Verification items for the finished model (mm, model axes). Face numbers are marked on the shaded views. Round coordinates to 2 decimals unless told otherwise and drop trailing zeros. Write each loop counter-clockwise with the first axis right and the second up, starting at its lowest first coordinate (ties: lowest second). Pieces come first, ordered by that corner, then holes. Notation, with made-up numbers: M 3.25,48 L 10.25,48 A12 cw 10.25,69 Z; hole C 78.5,18.25 d8. An arc over 180 degrees is marked long. One line per item, written item: value. Start each with the question number.
from build123d import *

# Parameters (mm, degrees)
F1_DEPTH      = 2
F3_DEPTH      = 2.2
F5_DEPTH      = 25
F6_R          = 1.5
F7_DEPTH      = 4.2
F8_R          = 2.75
F9_DEPTH      = 2
F10_S5_R      = 1.5
F10_T6_DEPTH  = 5
F10_S11_R     = 1.5
F10_T12_DEPTH = 5
F10_S17_R     = 1.5
F10_T18_DEPTH = 5
F10_S23_R     = 1.5
F10_T24_DEPTH = 5
F11_W         = 5.6
F11_H         = 2
F12_DEPTH     = 0.6
F13_T1_DEPTH  = 8.4722813233
F13_T3_DEPTH  = 8.4722813233
F14_SIZE      = 0.5


# Not quite as in the source:
# - a fillet or chamfer that OpenCascade refuses, or shapes differently, is made with other operations: its cross-section is extruded or revolved along the edge and cut away or added


with BuildPart() as f1:
    # F0 (on Top) → F1 (new body)
    with BuildSketch(Plane.XY):
        with BuildLine():
            Line((80, 0), (2, 0))
            ThreePointArc((2, 0), (0.5857864376, -0.5857864376), (0, -2))
            Line((0, -2), (0, -88))
            ThreePointArc((0, -88), (0.5857864376, -89.4142135624), (2, -90))
            Line((2, -90), (11.25, -90))
            Line((11.25, -90), (11.25, -62.5))
            Line((11.25, -62.5), (15.8564011104, -56.3307127986))
            ThreePointArc((15.8564011104, -56.3307127986), (16.5951030311, -54.9153368199), (16.85, -53.3392666362))
            Line((16.85, -53.3392666362), (16.85, -26))
            ThreePointArc((16.85, -26), (17.4357864376, -24.5857864376), (18.85, -24))
            Line((18.85, -24), (63.15, -24))
            ThreePointArc((63.15, -24), (64.5642135624, -24.5857864376), (65.15, -26))
            Line((65.15, -26), (65.15, -53.3392666362))
            ThreePointArc((65.15, -53.3392666362), (65.4048969689, -54.9153368199), (66.1435988896, -56.3307127986))
            Line((66.1435988896, -56.3307127986), (70.75, -62.5))
            Line((70.75, -62.5), (70.75, -90))
            Line((70.75, -90), (80, -90))
            ThreePointArc((80, -90), (81.4142135624, -89.4142135624), (82, -88))
            Line((82, -88), (82, -2))
            ThreePointArc((82, -2), (81.4142135624, -0.5857864376), (80, 0))
        make_face()
    extrude(amount=F1_DEPTH)

    # F2 (on face) → F3 (join)
    with BuildSketch(Plane(origin=(0, 0, 0), x_dir=(1, 0, 0), z_dir=(0, 0, -1))):
        with BuildLine():
            ThreePointArc((80, 0), (81.4142135624, 0.5857864376), (82, 2))
            Line((82, 2), (82, 88))
            ThreePointArc((82, 88), (81.4142135624, 89.4142135624), (80, 90))
            Line((80, 90), (70.75, 90))
            Line((70.75, 90), (70.75, 62.5))
            Line((70.75, 62.5), (70.75, 26))
            ThreePointArc((70.75, 26), (70.1642135624, 24.5857864376), (68.75, 24))
            Line((68.75, 24), (65.15, 24))
            Line((65.15, 24), (16.85, 24))
            Line((16.85, 24), (13.25, 24))
            ThreePointArc((13.25, 24), (11.8357864376, 24.5857864376), (11.25, 26))
            Line((11.25, 26), (11.25, 62.5))
            Line((11.25, 62.5), (11.25, 90))
            Line((11.25, 90), (2, 90))
            ThreePointArc((2, 90), (0.5857864376, 89.4142135624), (0, 88))
            Line((0, 88), (0, 2))
            ThreePointArc((0, 2), (0.5857864376, 0.5857864376), (2, 0))
            Line((2, 0), (80, 0))
        make_face()
    extrude(amount=F3_DEPTH)

    # F4 (on face) → F5 (cut)
    with BuildSketch(Plane.XY.offset(2)):
        with BuildLine():
            Line((18.3, -2), (10.5, -2))
            Line((10.5, -2), (10.5, -7.6))
            ThreePointArc((10.5, -7.6), (11.0857864376, -9.0142135624), (12.5, -9.6))
            Line((12.5, -9.6), (16.3, -9.6))
            ThreePointArc((16.3, -9.6), (17.7142135624, -9.0142135624), (18.3, -7.6))
            Line((18.3, -7.6), (18.3, -2))
        make_face()
    extrude(amount=-F5_DEPTH, mode=Mode.SUBTRACT)

    # F6 (on face) → F7 (cut)
    with BuildSketch(Plane.XY.offset(2)):
        with Locations((5.5, -84.5)):
            Circle(F6_R)
        with Locations((76.5, -84.5)):
            Circle(F6_R)
        with Locations((5.5, -5.5)):
            Circle(F6_R)
        with Locations((76.5, -5.5)):
            Circle(F6_R)
    extrude(amount=-F7_DEPTH, mode=Mode.SUBTRACT)

    # F8 (on face) → F9 (cut)
    with BuildSketch(Plane.XY.offset(2)):
        with Locations((5.5, -5.5)):
            Circle(F8_R)
        with Locations((76.5, -5.5)):
            Circle(F8_R)
        with Locations((76.5, -84.5)):
            Circle(F8_R)
        with Locations((5.5, -84.5)):
            Circle(F8_R)
    extrude(amount=-F9_DEPTH, mode=Mode.SUBTRACT)

    # F10: chamfer of 1.5 on 4 edges, made by hand


with BuildPart() as f10_tool2:
    # F10_s3 → F10_t4 (revolve)
    with BuildSketch(Plane.XZ.offset(84.5)):
        Polygon((8.25, 1.5), (6.75, 0), (8.25, 0), align=None)
    revolve(axis=Axis((5.5, -84.5, 0), (0, 0, 1)))

    # F10_s5 → F10_t6 (cut, symmetric)
    with BuildSketch(Plane.XY.offset(0.7)):
        with Locations((5.5, -84.5)):
            Circle(F10_S5_R)
    extrude(amount=F10_T6_DEPTH, both=True, mode=Mode.SUBTRACT)


with BuildPart() as f1_1:
    add(f1.part)

    # F10_t1: union F10_tool2
    add(f10_tool2.part)


with BuildPart() as f10_tool8:
    # F10_s9 → F10_t10 (revolve)
    with BuildSketch(Plane.XZ.offset(84.5)):
        Polygon((79.25, 1.5), (77.75, 0), (79.25, 0), align=None)
    revolve(axis=Axis((76.5, -84.5, 0), (0, 0, 1)))

    # F10_s11 → F10_t12 (cut, symmetric)
    with BuildSketch(Plane.XY.offset(0.7)):
        with Locations((76.5, -84.5)):
            Circle(F10_S11_R)
    extrude(amount=F10_T12_DEPTH, both=True, mode=Mode.SUBTRACT)


with BuildPart() as f1_2:
    add(f1_1.part)

    # F10_t7: union F10_tool8
    add(f10_tool8.part)


with BuildPart() as f10_tool14:
    # F10_s15 → F10_t16 (revolve)
    with BuildSketch(Plane.XZ.offset(5.5)):
        Polygon((8.25, 1.5), (6.75, 0), (8.25, 0), align=None)
    revolve(axis=Axis((5.5, -5.5, 0), (0, 0, 1)))

    # F10_s17 → F10_t18 (cut, symmetric)
    with BuildSketch(Plane.XY.offset(0.7)):
        with Locations((5.5, -5.5)):
            Circle(F10_S17_R)
    extrude(amount=F10_T18_DEPTH, both=True, mode=Mode.SUBTRACT)


with BuildPart() as f1_3:
    add(f1_2.part)

    # F10_t13: union F10_tool14
    add(f10_tool14.part)


with BuildPart() as f10_tool20:
    # F10_s21 → F10_t22 (revolve)
    with BuildSketch(Plane.XZ.offset(5.5)):
        Polygon((79.25, 1.5), (77.75, 0), (79.25, 0), align=None)
    revolve(axis=Axis((76.5, -5.5, 0), (0, 0, 1)))

    # F10_s23 → F10_t24 (cut, symmetric)
    with BuildSketch(Plane.XY.offset(0.7)):
        with Locations((76.5, -5.5)):
            Circle(F10_S23_R)
    extrude(amount=F10_T24_DEPTH, both=True, mode=Mode.SUBTRACT)


with BuildPart() as f1_4:
    add(f1_3.part)

    # F10_t19: union F10_tool20
    add(f10_tool20.part)

    # F11 (on face) → F12 (join)
    with BuildSketch(Plane(origin=(0, 0, 0), x_dir=(1, 0, 0), z_dir=(0, 0, -1))):
        with Locations((14.05, 43.5)):
            Rectangle(F11_W, F11_H)
        with Locations((67.95, 43.5)):
            Rectangle(F11_W, F11_H)
    extrude(amount=F12_DEPTH)

    # F13: fillet of radius 1.4 on 4 edges, made by hand

    # F13_s2 → F13_t1 (cut)
    with BuildSketch(Plane.YZ.offset(11.25)):
        with BuildLine():
            ThreePointArc((-42.5, 0), (-43.0008384595, -0.4409673646), (-43.6489125293, -0.6))
            Line((-43.6489125293, -0.6), (-42.5, -0.6))
            Line((-42.5, -0.6), (-42.5, 0))
        make_face()
        with BuildLine():
            ThreePointArc((-43.3510874707, -0.6), (-43.9991615405, -0.4409673646), (-44.5, 0))
            Line((-44.5, 0), (-44.5, -0.6))
            Line((-44.5, -0.6), (-43.3510874707, -0.6))
        make_face()
    extrude(amount=F13_T1_DEPTH, mode=Mode.SUBTRACT)

    # F13_s4 → F13_t3 (cut)
    with BuildSketch(Plane.YZ.offset(62.2777186767)):
        with BuildLine():
            ThreePointArc((-43.6489125293, -0.6), (-43.0008384595, -0.4409673646), (-42.5, 0))
            Line((-42.5, 0), (-42.5, -0.6))
            Line((-42.5, -0.6), (-43.6489125293, -0.6))
        make_face()
        with BuildLine():
            ThreePointArc((-44.5, 0), (-43.9991615405, -0.4409673646), (-43.3510874707, -0.6))
            Line((-43.3510874707, -0.6), (-44.5, -0.6))
            Line((-44.5, -0.6), (-44.5, 0))
        make_face()
    extrude(amount=F13_T3_DEPTH, mode=Mode.SUBTRACT)

    # F14
    f14_edges = [f1_4.edges().sort_by_distance(p)[0] for p in [
        (0.585786, -0.585786, 2),
        (41, 0, 2),
        (0, -45, 2),
        (10.5, -4.8, 2),
        (14.4, -2, 2),
        (18.3, -4.8, 2),
        (17.714214, -9.014214, 2),
        (14.4, -9.6, 2),
        (11.085786, -9.014214, 2),
        (81.414214, -0.585786, 2),
        (82, -45, 2),
        (11.25, -76.25, 2),
        (6.625, -90, 2),
        (0.585786, -89.414214, 2),
        (81.414214, -89.414214, 2),
        (75.375, -90, 2),
        (70.75, -76.25, 2),
        (68.446799, -59.415356, 2),
        (65.404897, -54.915337, 2),
        (65.15, -39.669633, 2),
        (64.564214, -24.585786, 2),
        (41, -24, 2),
        (17.435786, -24.585786, 2),
        (16.85, -39.669633, 2),
        (16.595103, -54.915337, 2),
        (13.553201, -59.415356, 2),
    ]]
    chamfer(f14_edges, length=F14_SIZE)


solid = f1_4.part
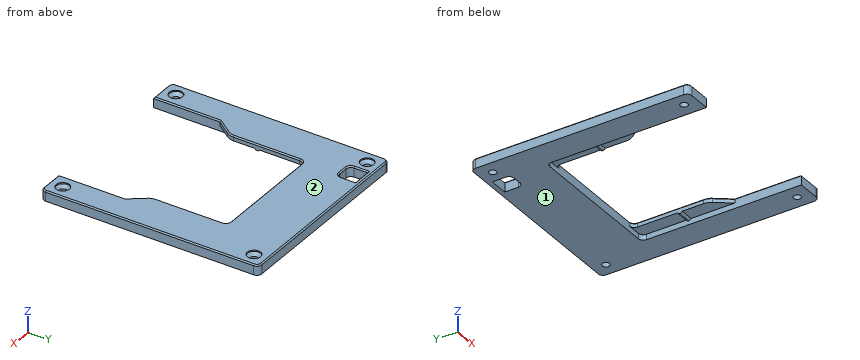
1) Cross-section at A-A (y = -84.5). Record the boundary of the cut face in (x, z).
2) Cross-section at C-C (x = 76.5). Record the boundary of the cut face in (y, z).
3) Cross-section at D-D (y = -5.5). Record the boundary of the cut face in (x, z), then the cut area to 3 significant figures.
4) Thickness scan on line 1 (X direction, y = -84.5, z = -1.3); line 2 (Y direction, x = 76.5, z = -0.4); line 3 (X direction, y = -74, z = 0.55). Record the ranges inside material, lowest first.
5) Cross-section at B-B (y = -30). Record the boundary of the cut face in (x, z), then the cut area to 3 significant figures.
6) Gauge pin test, flat ends, axial feed: pin 1 Ø4.5 at (x, y) = (5.5, -5.5) entering from +Z; pin 2 Ø3 at (x, y) = (67.5, -50) entering from -Z; pin 3 Ø2.5 at (x, y) = (76.5, -5.5) entering from -Z; pin 4 Ø5 at (x, y) = (5.5, -5.5) entering from +Z. Record the tip position at first contact, or that the pin passes through.
7) Mould release check, pull along Z, two halves, no side actions. Record for the marked faces 1 and 2: pulls with the +Z half, pulls with the -Z half, needs draft (parallel to the pull), parting line crosses it, or undercut.
Results below:
1. outline: M 0,-2.2 L 4,-2.2 L 4,0.25 L 2.75,1.5 L 2.75,2 L 0.5,2 L 0,1.5 Z; M 7,-2.2 L 11.25,-2.2 L 11.25,1.5 L 10.75,2 L 8.25,2 L 8.25,1.5 L 7,0.25 Z; M 70.75,-2.2 L 75,-2.2 L 75,0.25 L 73.75,1.5 L 73.75,2 L 71.25,2 L 70.75,1.5 Z; M 78,-2.2 L 82,-2.2 L 82,1.5 L 81.5,2 L 79.25,2 L 79.25,1.5 L 78,0.25 Z
2. outline: M -90,-2.2 L -86,-2.2 L -86,0.25 L -87.25,1.5 L -87.25,2 L -89.5,2 L -90,1.5 Z; M -83,-2.2 L -7,-2.2 L -7,0.25 L -8.25,1.5 L -8.25,2 L -81.75,2 L -81.75,1.5 L -83,0.25 Z; M -4,-2.2 L 0,-2.2 L 0,1.5 L -0.5,2 L -2.75,2 L -2.75,1.5 L -4,0.25 Z
3. outline: M 0,-2.2 L 4,-2.2 L 4,0.25 L 2.75,1.5 L 2.75,2 L 0.5,2 L 0,1.5 Z; M 7,-2.2 L 10.5,-2.2 L 10.5,1.5 L 10,2 L 8.25,2 L 8.25,1.5 L 7,0.25 Z; M 18.3,-2.2 L 75,-2.2 L 75,0.25 L 73.75,1.5 L 73.75,2 L 18.8,2 L 18.3,1.5 Z; M 78,-2.2 L 82,-2.2 L 82,1.5 L 81.5,2 L 79.25,2 L 79.25,1.5 L 78,0.25 Z
3. area: 280 mm²
4. line 1: x = 0 to 4, 7 to 11.25, 70.75 to 75, 78 to 82
4. line 2: y = -90 to -86, -83 to -7, -4 to 0
4. line 3: x = 0 to 11.25, 70.75 to 82
5. outline: M 0,-2.2 L 11.25,-2.2 L 11.25,0 L 16.85,0 L 16.85,1.5 L 16.35,2 L 0.5,2 L 0,1.5 Z; M 65.15,0 L 70.75,0 L 70.75,-2.2 L 82,-2.2 L 82,1.5 L 81.5,2 L 65.65,2 L 65.15,1.5 Z
5. area: 116 mm²
6. pin 1: stops at z = 1
6. pin 2: stops at z = 0
6. pin 3: passes through
6. pin 4: stops at z = 1.25
7. face 1: pulls with the -Z half
7. face 2: pulls with the +Z half
